from build123d import *

# Parameters (mm, degrees)
SKETCH1_R                               = 84.93125
BOSS_EXTRUDE1_DEPTH                     = 25.4
CBORE_FOR_M6_HEX_HEAD_BOLT1_D           = 7
CBORE_FOR_M6_HEX_HEAD_BOLT1_CBORE_D     = 14.547
CBORE_FOR_M6_HEX_HEAD_BOLT1_CBORE_DEPTH = 4


with BuildPart() as part:
    # Sketch1 → Boss-Extrude1 (new body)
    with BuildSketch(Plane.XY):
        with BuildLine():
            ThreePointArc((-76.246005737, 105.719498865), (-39.105377809, 92.490752346), (0, 87.47125))
            ThreePointArc((0, 87.47125), (39.105377809, 92.490752346), (76.246005737, 105.719498865))
            ThreePointArc((76.246005737, 105.719498865), (102.262666579, 102.262666579), (105.719498865, 76.246005737))
            ThreePointArc((105.719498865, 76.246005737), (92.490752346, 39.105377809), (87.47125, 0))
            ThreePointArc((87.47125, 0), (92.490752346, -39.105377809), (105.719498865, -76.246005737))
            ThreePointArc((105.719498865, -76.246005737), (102.262666579, -102.262666579), (76.246005737, -105.719498865))
            ThreePointArc((76.246005737, -105.719498865), (39.105377809, -92.490752346), (0, -87.47125))
            ThreePointArc((0, -87.47125), (-39.105377809, -92.490752346), (-76.246005737, -105.719498865))
            ThreePointArc((-76.246005737, -105.719498865), (-102.262666579, -102.262666579), (-105.719498865, -76.246005737))
            ThreePointArc((-105.719498865, -76.246005737), (-92.490752346, -39.105377809), (-87.47125, 0))
            ThreePointArc((-87.47125, 0), (-92.490752346, 39.105377809), (-105.719498865, 76.246005737))
            ThreePointArc((-105.719498865, 76.246005737), (-102.262666579, 102.262666579), (-76.246005737, 105.719498865))
        make_face()
        Circle(SKETCH1_R, mode=Mode.SUBTRACT)
    extrude(amount=BOSS_EXTRUDE1_DEPTH)

    # CBORE for M6 Hex Head Bolt1 (through all)
    with Locations(Plane(origin=(0, 0, 0), x_dir=(-1, 0, 0), z_dir=(0, 0, -1))):
        with Locations((-86.996231173, 86.996231173), (86.996231173, 86.996231173), (86.996231173, -86.996231173), (-86.996231173, -86.996231173)):
            CounterBoreHole(CBORE_FOR_M6_HEX_HEAD_BOLT1_D / 2, CBORE_FOR_M6_HEX_HEAD_BOLT1_CBORE_D / 2, CBORE_FOR_M6_HEX_HEAD_BOLT1_CBORE_DEPTH)


solid = part.part
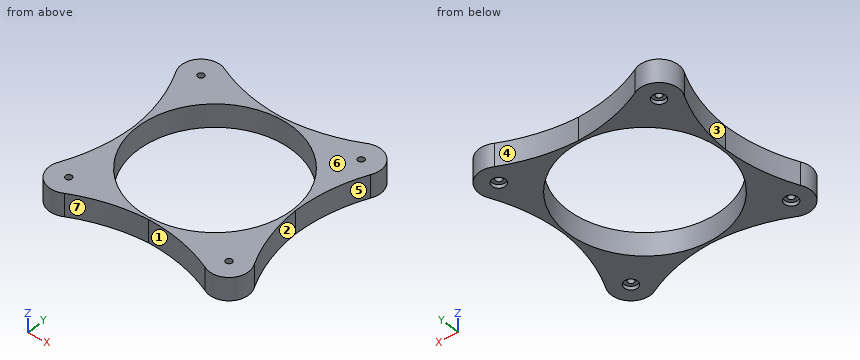
The model under review builds one solid part; all positions refer to its coordinate system, in mm. Face numbers are marked on the shaded views. A direction names the side the tool comes from. Give positions to 0.01 mm unless a question says otherwise; leave off trailing zeros. Loops run counter-clockwise (first coordinate to the right, second up) from the corner with the lowest first, then second, coordinate; pieces in that order, holes last. Notation, with made-up numbers: (53.25, 50.5) -> (104.25, 50.5) arc R24 ccw to (104.25, 88.5) -> close; hole circle Ø5 at (-7.75, 72). An arc over 180 degrees is marked (long way). Answer as a JSON object with one key per item and string values. Group by question number.
Q1. Draft analysis for pull direction X (two halves, no side actions). For the marked faces 5, 6 and 7, state which applies: pulls with the +X half, pulls with the -X half, needs draft (parallel to the pull), parting line crosses it, or undercut.
Q2. Insertion check: pin 1 (11.5 mm diameter, centred on x = -87, y = -87, fed in from +Z); pin 2 (13 mm diameter, centred on x = 87, y = 87, fed in from -Z); pin 3 (3 mm diameter, centred on y = 41.5, z = 14, fed in from -X); pin 4 (2 mm diameter, centred on y = -60, z = 7.5, fed in from -X). Each pin has a flat end and moves straight along its axis. Give the tip position at first contact, or say it passes through.
Q3. Wall thickness on line 1 along X through (y, z) = (85.5, 16); line 2 along X through (y, z) = (12, 16); line 3 along Y through (x, z) = (52, 8): over which ranges is each line inside the solid? List them lowest first.
Q4. Tool access review of the marked faces 1, 2, 3 and 4: name each direction out of +Z, -Z, +X, -X, +Y, -Y from which nothing blocks a thin tool from reaching the whole face with its end or side.
Q5. Take a section at C-C (z = 19.5). Write out the cut boundary in (x, y).
Q6. Take a section at A-A (x = 43). Write out the cut boundary in (y, z).
Q7. Take a section at B-B (y = -9.5). Write out the cut boundary in (x, z).
Answer below:
{
 "1": {"face 5": "pulls with the +X half", "face 6": "needs draft", "face 7": "undercut"},
 "2": {"pin 1": "stops at z = 25.4", "pin 2": "stops at z = 4", "pin 3": "stops at x = -93.47", "pin 4": "stops at x = -99.19"},
 "3": {"line 1": "x = -108.53 to -90.16, -83.83 to 83.83, 90.16 to 108.53", "line 2": "x = -88.11 to -84.08, 84.08 to 88.11", "line 3": "y = -96.08 to -67.15, 67.15 to 96.08"},
 "4": {"face 1": "+Z, -Z, -Y", "face 2": "+Z, -Z, +X", "face 3": "+Z, -Z, -X", "face 4": "+Z, -Z, +Y"},
 "5": {"outline": "(-105.72, -76.25) arc R21.59 ccw to (-76.25, -105.72) arc R184.15 cw to (0, -87.47) arc R184.15 cw to (76.25, -105.72) arc R21.59 ccw to (105.72, -76.25) arc R184.15 cw to (87.47, 0) arc R184.15 cw to (105.72, 76.25) arc R21.59 ccw to (76.25, 105.72) arc R184.15 cw to (0, 87.47) arc R184.15 cw to (-76.25, 105.72) arc R21.59 ccw to (-105.72, 76.25) arc R184.15 cw to (-87.47, 0) arc R184.15 cw to start; hole circle Ø7 at (-87, -87); hole circle Ø7 at (-87, 87); hole circle Ø169.86 at (0, 0); hole circle Ø7 at (87, -87); hole circle Ø7 at (87, 87)"},
 "6": {"outline": "(-93.47, 0) -> (-73.24, 0) -> (-73.24, 25.4) -> (-93.47, 25.4) -> close; (73.24, 0) -> (93.47, 0) -> (93.47, 25.4) -> (73.24, 25.4) -> close"},
 "7": {"outline": "(-87.91, 0) -> (-84.4, 0) -> (-84.4, 25.4) -> (-87.91, 25.4) -> close; (84.4, 0) -> (87.91, 0) -> (87.91, 25.4) -> (84.4, 25.4) -> close"}
}
